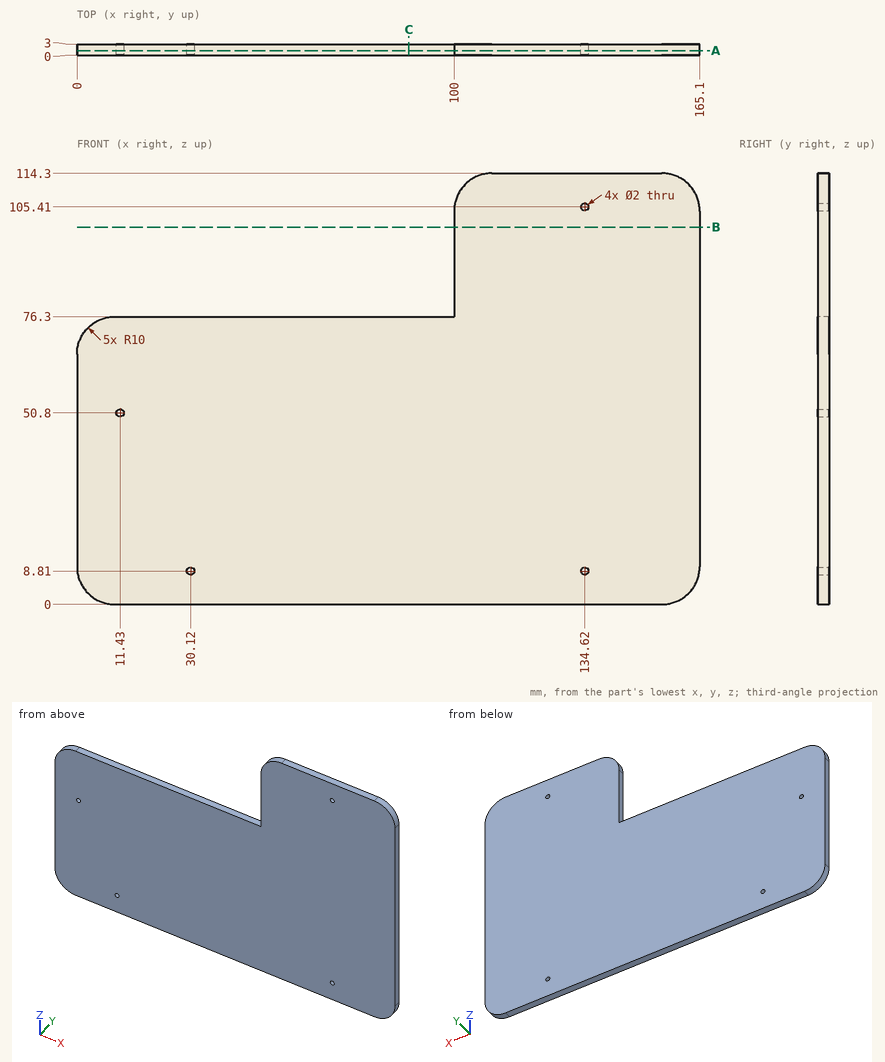
Study the drawing (mm; zero at the part's minimum x, y, z) and answer. Give positions to 0.01 mm unless a question says otherwise; leave off trailing zeros. Loops run counter-clockwise (first coordinate to the right, second up) from the corner with the lowest first, then second, coordinate; pieces in that order, holes last. Notation, with made-up numbers: M 69.25,40.25 L 104.25,40.25 A34 ccw 104.25,74.25 Z; hole C 23.5,3.25 d11. An arc over 180 degrees is marked long. One line per item, written item: value.
1. Section B-B on z = 100 is taken. Determine the outline of the cut face in (x, y), plus the area to 3 significant figures.
Found:
outline: M 100,0 L 165.1,0 L 165.1,3 L 100,3 Z
area: 195 mm^2
2. Each of these flat-tipped pins is pushed along its axis until it touches: P1, Ø1.5, axis at x = 37.5, y = 1.5, coming from the +Z side; P2, Ø1.8, axis at x = 11.43, z = 50.8, coming from the +Y side. Where does it stop, or does it pass through?
Found:
P1: z = 76.3
P2: through
3. Section A-A on y = 1.25 is taken. Determine the outline of the cut face in (x, z), plus the area to 3 significant figures.
Found:
outline: M 0,10 A10 ccw 10,0 L 155.1,0 A10 ccw 165.1,10 L 165.1,104.3 A10 ccw 155.1,114.3 L 110,114.3 A10 ccw 100,104.3 L 100,76.3 L 10,76.3 A10 ccw 0,66.3 Z; hole C 11.43,50.8 d2; hole C 30.12,8.81 d2; hole C 134.62,8.81 d2; hole C 134.62,105.41 d2
area: 15,000 mm^2
4. Section C-C on x = 88 is taken. Determine the outline of the cut face in (y, z), plus the area to 3 significant figures.
Found:
outline: M 0,0 L 3,0 L 3,76.3 L 0,76.3 Z
area: 229 mm^2
5. Find the intervals of material crossed by probe 1 along Z at (x, y) = (134.62, 1.4); probe 2 along X at (y, z) = (0.9, 50.8); probe 3 along Z at (x, y) = (11.43, 2.1), in increasing order.
Found:
probe 1: 0 to 7.81, 9.81 to 104.41, 106.41 to 114.3
probe 2: 0 to 10.43, 12.43 to 165.1
probe 3: 0 to 49.8, 51.8 to 76.3
